from build123d import *

# Parameters (mm, degrees)
SKETCH_1_W                   = 140
SKETCH_1_H                   = 25
EXTRUDE_1_DEPTH              = 40
SKETCH_2_W                   = 104
SKETCH_2_H                   = 34
CUT_EXTRUDE_1_DEPTH          = 85.409715081
SKETCH_3_W                   = 17.5
SKETCH_3_H                   = 21
CUT_EXTRUDE_2_DEPTH          = 25
HOLE_WIZARD_M6_1_D           = 8
HOLE_WIZARD_M6_1_CBORE_D     = 15
HOLE_WIZARD_M6_1_CBORE_DEPTH = 6.4
FILLET_1_R                   = 1
FILLET_2_R                   = 1


with BuildPart() as part:
    # 草图1 → 凸台-拉伸1 (new body)
    with BuildSketch(Plane(origin=(0, 0, 0), x_dir=(1, 0, 0), z_dir=(0, 1, 0))):
        Rectangle(SKETCH_1_W, SKETCH_1_H)
    extrude(amount=EXTRUDE_1_DEPTH)

    # 草图2 → 切除-拉伸1 (cut, through all)
    with BuildSketch(Plane.XY.offset(12.5)):
        with Locations((0, 17)):
            Rectangle(SKETCH_2_W, SKETCH_2_H)
        Polygon((-70, 40), (-50, 40), (-70, 18), align=None)
        Polygon((70, 40), (50, 40), (70, 18), align=None)
    extrude(amount=-CUT_EXTRUDE_1_DEPTH, mode=Mode.SUBTRACT)

    # 草图3 → 切除-拉伸2 (cut)
    with BuildSketch(Plane(origin=(0, 40, 0), x_dir=(1, 0, 0), z_dir=(0, 1, 0))):
        with Locations((-61.25, 0)):
            Rectangle(SKETCH_3_W, SKETCH_3_H)
        with Locations((61.25, 0)):
            Rectangle(SKETCH_3_W, SKETCH_3_H)
    extrude(amount=-CUT_EXTRUDE_2_DEPTH, mode=Mode.SUBTRACT)

    # M6 六角凹头螺钉的柱形沉头孔1 (through all)
    with Locations(Plane(origin=(0, 15, 0), x_dir=(-1, 0, 0), z_dir=(0, 1, 0))):
        with Locations((60, 0), (-60, 0)):
            CounterBoreHole(HOLE_WIZARD_M6_1_D / 2, HOLE_WIZARD_M6_1_CBORE_D / 2, HOLE_WIZARD_M6_1_CBORE_DEPTH)

    # 圆角1
    fillet_1_edges = [part.edges().sort_by_distance(p)[0] for p in [
        (-52, 17, -12.5),
        (-52, 0, 0),
        (0, 34, -12.5),
        (-52, 34, 0),
        (52, 17, -12.5),
        (52, 34, 0),
        (52, 0, 0),
        (-52, 17, 12.5),
        (52, 17, 12.5),
        (0, 34, 12.5),
    ]]
    fillet(fillet_1_edges, radius=FILLET_1_R)

    # 圆角2
    fillet_2_edges = [part.edges().sort_by_distance(p)[0] for p in [
        (0, 40, 12.5),
        (-70, 9, -12.5),
        (-70, 9, 12.5),
        (-60, 29, -12.5),
        (-60, 29, 12.5),
        (0, 40, -12.5),
        (70, 9, -12.5),
        (70, 9, 12.5),
        (60, 29, -12.5),
        (60, 29, 12.5),
    ]]
    fillet(fillet_2_edges, radius=FILLET_2_R)


solid = part.part
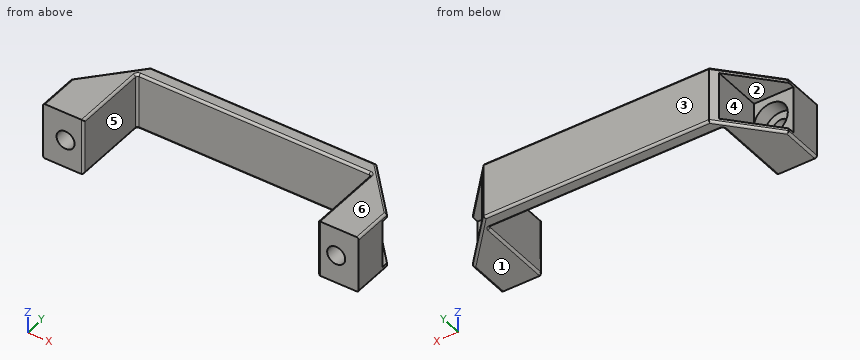
Check sheet for the modelled part. Datum: model origin and axes. Units: mm. Face numbers are marked on the shaded views. A direction names the side the tool comes from. Give positions to 0.01 mm unless a question says otherwise; leave off trailing zeros. Loops run counter-clockwise (first coordinate to the right, second up) from the corner with the lowest first, then second, coordinate; pieces in that order, holes last. Notation, with made-up numbers: M -17,25 L 16,25 A22 cw 16,42 Z; hole C 1.5,16.5 d9. An arc over 180 degrees is marked long. Use a Markdown table: item, result. Add a question column.
Q1. Scan lines: line 1 along X through (y, z) = (2.5, -5.75); line 2 along X through (y, z) = (28, 4.5); line 3 along Z through (x, y) = (60, 12). Record each from-to range of solid material in increasing order. Write a range as [from, to].
Q2. Mould release check, pull along Z, two halves, no side actions. Record for the marked faces 1, 2 and 3: pulls with the +Z half, pulls with the -Z half, needs draft (parallel to the pull), parting line crosses it, or undercut.
Q3. Sectioned sample at B-B, the plane z = -6. Record the cut outline in (x, y), then the cut area to 3 significant figures.
Q4. Sectioned sample at C-C, the plane x = -18. Record the cut outline in (y, z).
Q5. Go/stop test with flat-tipped pins: pin 1 (12 mm diameter, centred on x = 63, z = -1, fed in from +Y); pin 2 (6.5 mm diameter, centred on x = -60, z = 0, fed in from +Y); pin 3 (9 mm diameter, centred on x = 60, z = 0, fed in from +Y); pin 4 (14 mm diameter, centred on x = 58, z = -3, fed in from +Y). Record where each tip stops, or that it passes through.
Q6. Tool access check on the marked faces 4, 5 and 6. Record the directions out of +Z, -Z, +X, -X, +Y, -Y that give a thin tool (end or side, any length) a straight path to the whole face; none if there is none.
Q7. Sectioned sample at A-A, the plane y = 11.5. Record the cut outline in (x, z).
Verdict:
| question | item | result |
|---|---|---|
| 1 | line 1 | [-70, -52], [52, 70] |
| 1 | line 2 | [-52.5, -52], [52, 52.5] |
| 1 | line 3 | [-12.5, -7.5], [7.5, 12.5] |
| 2 | face 1 | pulls with the -Z half |
| 2 | face 2 | undercut |
| 2 | face 3 | needs draft |
| 3 | outline | M -70,0 L -53,0 A1 ccw -52,1 L -52,33 A1 cw -51,34 L 51,34 A1 cw 52,33 L 52,1 A1 ccw 53,0 L 70,0 L 70,15 L 64.5,15 L 64.5,8.6 L 55.5,8.6 L 55.5,15 L 52.5,15 L 52.5,37.25 L 50,40 L -50,40 L -52.5,37.25 L -52.5,15 L -55.5,15 L -55.5,8.6 L -64.5,8.6 L -64.5,15 L -70,15 Z |
| 3 | area | 1,070 mm^2 |
| 4 | outline | M 34,-11.5 A1 ccw 35,-12.5 L 39,-12.5 A1 ccw 40,-11.5 L 40,11.5 A1 ccw 39,12.5 L 35,12.5 A1 ccw 34,11.5 Z |
| 5 | pin 1 | y = 15 |
| 5 | pin 2 | through |
| 5 | pin 3 | y = 8.6 |
| 5 | pin 4 | y = 38.9 |
| 6 | face 4 | -X, +Y |
| 6 | face 5 | +Z, -Z, -Y |
| 6 | face 6 | +Z, +X, -X, +Y, -Y |
| 7 | outline | M -70,-11.5 A1 ccw -69,-12.5 L -53,-12.5 A1 ccw -52,-11.5 L -52,11.5 A1 ccw -53,12.5 L -69,12.5 A1 ccw -70,11.5 Z; M 52,-11.5 A1 ccw 53,-12.5 L 69,-12.5 A1 ccw 70,-11.5 L 70,11.5 A1 ccw 69,12.5 L 53,12.5 A1 ccw 52,11.5 Z; hole C -60,0 d15; hole C 60,0 d15 |
